Geometry check sheet. Reference: the model listing, model coordinates, mm. A direction names the side the tool comes from. Round coordinates to 2 decimals unless told otherwise and drop trailing zeros. Loops run counter-clockwise (first coordinate to the right, second up) from the corner with the lowest first, then second, coordinate; pieces in that order, holes last. Notation, with made-up numbers: (8, -30.5) -> (30, -30.5) arc R11 ccw to (30, -19.5) -> close; hole circle Ø7 at (40, -39). An arc over 180 degrees is marked (long way). Use a Markdown table: item, result. Add a question column.
Q1. Sectioned sample at A-A, the plane x = 0. Enter the section's corners in (y, z).
Q2. Sectioned sample at D-D, the plane y = 1. Enter the section's corners in (x, z) (3 decimals), then the cut area to 3 significant figures.
Q3. Sectioned sample at B-B, the plane z = -6. Enter the section's corners in (x, y), then the cut area to 3 significant figures.
Q4. Gauge pin test, flat ends, axial feed: P1, Ø5, axis at x = 7.5, y = -4.5, coming from the -Z side (3 decimals); P2, Ø4, axis at y = -14.5, z = 7, coming from the +X side (3 decimals); P3, Ø5, axis at x = 5, y = -10, coming from the +Z side. Record the tip position at first contact, or that the pin passes through.
Q5. Sectioned sample at C-C, the plane z = 10.5. Enter the section's corners in (x, y), then the cut area to 3 significant figures.
Q6. Material ranges on L1, parallel to Z at x = -9, y = 1.25; L2, parallel to X at y = 1.1, z = -4.75; L3, parallel to Y at x = 3.75, z = 9.75, recorded low to high.
Q7. Release check for a two-part mould opening along X. For faces 6 (the face through (0, 3, -5)), 7 (the face through (9.619, 0.986, 3.863)), 8 (the face through (7.65, -9.86, -2.34)), 9 (the face through (-4.31, 2.838, -2.535)) record: released by +X, released by -X, zero draft, split by the parting line, or undercut.
Q8. Set-up check for faces 1 (the face through (0, 3, 5)), 2 (the face through (4.31, 2.838, 2.535)), 3 (the face through (4.35, 2.838, -2.465)), 4 (the face through (-4.35, 2.838, 2.465)), 5 (the face through (0.45, 2.86, 1.43)): record each of +Z, -Z, +X, -X, +Y, -Y from which the full face is reachable in a straight line by a thin tool's end or side.
```python
from build123d import *

# Parameters (mm, degrees)
SKETCH_1_R               = 12.5
EXTRUDE_1_DEPTH          = 2
SKETCH_2_R               = 1.65
CUT_EXTRUDE_1_DEPTH      = 18.790446875
PATTERN_CIRCULAR_1_COUNT = 6
SKETCH_3_R               = 8
EXTRUDE_2_DEPTH          = 20
EXTRUDE_3_DEPTH          = 1.7
SKETCH_5_R               = 3
SKETCH_5_R_2             = 1.5
CUT_EXTRUDE_2_DEPTH      = 1.7


with BuildPart() as part:
    # Эскиз1 → Бобышка-Вытянуть1 (new body)
    with BuildSketch(Plane(origin=(0, 0, 0), x_dir=(1, 0, 0), z_dir=(0, 1, 0))):
        with Locations(Location((0, 0, 0), (0, 0, 270))):
            Circle(SKETCH_1_R)
    extrude(amount=EXTRUDE_1_DEPTH)

    # Эскиз2 → Вырез-Вытянуть1 (cut, through all)
    with BuildSketch(Plane.XZ):
        with Locations(Location((0, -9.5, 0), (0, 0, 270))):
            Circle(SKETCH_2_R)
    cut_extrude_1 = extrude(amount=-CUT_EXTRUDE_1_DEPTH, mode=Mode.SUBTRACT)

    # Круговой массив1: Вырез-Вытянуть1 ×6 about axis
    pattern_circular_1_axis = Axis((0, 0, 0), (0, 1, 0))
    for i in range(1, PATTERN_CIRCULAR_1_COUNT):
        add(cut_extrude_1.rotate(pattern_circular_1_axis, i * 360 / PATTERN_CIRCULAR_1_COUNT), mode=Mode.SUBTRACT)

    # Эскиз3 → Бобышка-Вытянуть2 (add)
    with BuildSketch(Plane.XZ):
        with Locations(Location((0, 0, 0), (0, 0, 85.481135603))):
            Circle(SKETCH_3_R)
    extrude(amount=EXTRUDE_2_DEPTH)

    # Эскиз4 → Бобышка-Вытянуть3 (add)
    with BuildSketch(Plane(origin=(0, 2, 0), x_dir=(1, 0, 0), z_dir=(0, 1, 0))):
        Polygon((-5.773502692, 0), (-2.886751346, -5), (2.886751346, -5), (5.773502692, 0), (2.886751346, 5), (-2.886751346, 5), align=None)
    extrude(amount=EXTRUDE_3_DEPTH)

    # Эскиз5 → Вырез-Вытянуть2 (cut)
    with BuildSketch(Plane(origin=(0, 3.7, 0), x_dir=(1, 0, 0), z_dir=(0, 1, 0))):
        with Locations(Location((0, 0, 0), (0, 0, 270))):
            Circle(SKETCH_5_R)
        with Locations(Location((0, 0, 0), (0, 0, 270))):
            Circle(SKETCH_5_R_2, mode=Mode.SUBTRACT)
    extrude(amount=-CUT_EXTRUDE_2_DEPTH, mode=Mode.SUBTRACT)


solid = part.part
```
Values:
| question | item | result |
|---|---|---|
| 1 | outline | (-20, -8) -> (0, -8) -> (0, -7.85) -> (2, -7.85) -> (2, -5) -> (3.7, -5) -> (3.7, -3) -> (2, -3) -> (2, -1.5) -> (3.7, -1.5) -> (3.7, 1.5) -> (2, 1.5) -> (2, 3) -> (3.7, 3) -> (3.7, 5) -> (2, 5) -> (2, 7.85) -> (0, 7.85) -> (0, 8) -> (-20, 8) -> close; (0, -12.5) -> (2, -12.5) -> (2, -11.15) -> (0, -11.15) -> close; (0, 11.15) -> (2, 11.15) -> (2, 12.5) -> (0, 12.5) -> close |
| 2 | outline | circle Ø25 at (0, 0); hole circle Ø3.3 at (-8.227, -4.75); hole circle Ø3.3 at (-8.227, 4.75); hole circle Ø3.3 at (0, -9.5); hole circle Ø3.3 at (0, 9.5); hole circle Ø3.3 at (8.227, -4.75); hole circle Ø3.3 at (8.227, 4.75) |
| 2 | area | 440 mm^2 |
| 3 | outline | (-10.97, 0) -> (-9.3, 0) -> (-9.3, 2) -> (-10.97, 2) -> close; (-7.15, 0) -> (-5.29, 0) -> (-5.29, -20) -> (5.29, -20) -> (5.29, 0) -> (7.15, 0) -> (7.15, 2) -> (-7.15, 2) -> close; (9.3, 0) -> (10.97, 0) -> (10.97, 2) -> (9.3, 2) -> close |
| 3 | area | 247 mm^2 |
| 4 | P1 | z = -6.245 |
| 4 | P2 | x = 6.245 |
| 4 | P3 | z = 7.6 |
| 5 | outline | (-6.78, 0) -> (-1.31, 0) -> (-1.31, 2) -> (-6.78, 2) -> close; (1.31, 0) -> (6.78, 0) -> (6.78, 2) -> (1.31, 2) -> close |
| 5 | area | 21.9 mm^2 |
| 6 | L1 | -8.67 to -6.21, -3.29 to 3.29, 6.21 to 8.67 |
| 6 | L2 | -11.56 to -9.88, -6.58 to 6.58, 9.88 to 11.56 |
| 6 | L3 | 0 to 2 |
| 7 | face 6 | zero draft |
| 7 | face 7 | undercut |
| 7 | face 8 | split by the parting line |
| 7 | face 9 | released by -X |
| 8 | face 1 | +Z, +X, -X, +Y |
| 8 | face 2 | +Z, +X, +Y |
| 8 | face 3 | -Z, +X, +Y |
| 8 | face 4 | +Z, -X, +Y |
| 8 | face 5 | +Y |
